Build history of the part. All positions in model axes, mm. A direction names the side the tool comes from. Round coordinates to 2 decimals unless told otherwise and drop trailing zeros. Write each loop counter-clockwise with the first axis right and the second up, starting at its lowest first coordinate (ties: lowest second). Pieces come first, ordered by that corner, then holes.
from build123d import *

# Parameters (mm, degrees)
SKETCH_1_W          = 135
SKETCH_1_H          = 80
EXTRUDE_1_DEPTH     = 60
CUT_EXTRUDE_START   = -1.5
CUT_EXTRUDE_1_DEPTH = 57
CUT_EXTRUDE_2_REACH = 170.003
SKETCH_4_R          = 23.5
SKETCH_5_W          = 135
SKETCH_5_H          = 15
EXTRUDE_2_DEPTH     = 5
M5_C_1_D            = 5.3
M5_C_1_DEPTH        = 5.2
M5_C_1_CBORE_D      = 11
M5_C_1_CBORE_DEPTH  = 0.5
M5_C_1_TIP          = 1.59228064
FILLET_1_R          = 5
FILLET_2_R          = 5
FILLET_3_R          = 5


with BuildPart() as part:
    # 草图1 → 凸台-拉伸1 (new body)
    with BuildSketch(Plane.XY):
        with Locations((67.5, -40)):
            Rectangle(SKETCH_1_W, SKETCH_1_H)
    extrude(amount=EXTRUDE_1_DEPTH)

    # 草图2 → 切除-拉伸1 (cut)
    with BuildSketch(Plane.XY.offset(60).offset(CUT_EXTRUDE_START)):
        Polygon((24.108601621, -76.68), (13.8, -76.68), (13.8, -19.68), (68.3, -19.68), (68.3, -76.68), align=None)
    extrude(amount=-CUT_EXTRUDE_1_DEPTH, mode=Mode.SUBTRACT)

    # 草图4 → 切除-拉伸2 (cut, up to next)
    with BuildSketch(Plane(origin=(135, 0, 0), x_dir=(0, 0, -1), z_dir=(1, 0, 0)), mode=Mode.PRIVATE) as cut_extrude_2_sk1:
        with Locations(Location((-30, -48.18, 0), (0, 0, 90))):
            Circle(SKETCH_4_R)
    cut_extrude_2_tool1 = extrude(cut_extrude_2_sk1.sketch, amount=-CUT_EXTRUDE_2_REACH, mode=Mode.PRIVATE) & part.part
    add(cut_extrude_2_tool1.solids().sort_by_distance((135, -48.18, 30))[0], mode=Mode.SUBTRACT)

    # 草图5 → 凸台-拉伸2 (add)
    with BuildSketch(Plane(origin=(0, 0, 0), x_dir=(1, 0, 0), z_dir=(0, 1, 0))):
        with Locations((67.5, 7.5)):
            Rectangle(SKETCH_5_W, SKETCH_5_H)
        with Locations((67.5, -67.5)):
            Rectangle(SKETCH_5_W, SKETCH_5_H)
    extrude(amount=-EXTRUDE_2_DEPTH)

    # M5 六角头螺栓C级的柱形沉头孔1
    with Locations(Plane(origin=(0, -5, 0), x_dir=(-1, 0, 0), z_dir=(0, -1, 0))):
        with Locations((-110, 7.5), (-25, 7.5), (-110, -67.5), (-25, -67.5)):
            CounterBoreHole(M5_C_1_D / 2, M5_C_1_CBORE_D / 2, M5_C_1_CBORE_DEPTH, depth=M5_C_1_DEPTH)
            with Locations((0, 0, -(M5_C_1_DEPTH + M5_C_1_TIP / 2))):  # 118° drill point
                Cone(0, M5_C_1_D / 2, M5_C_1_TIP, mode=Mode.SUBTRACT)

    # 圆角1
    fillet_1_edges = [part.edges().sort_by_distance(p)[0] for p in [
        (0, -42.5, 0),
        (0, -42.5, 60),
    ]]
    fillet(fillet_1_edges, radius=FILLET_1_R)

    # 圆角2
    fillet_2_edges = [part.edges().sort_by_distance(p)[0] for p in [
        (70, -80, 60),
        (70, -80, 0),
        (0, -80, 30),
        (1.464466094, -80, 1.464466094),
        (1.464466094, -80, 58.535533906),
    ]]
    fillet(fillet_2_edges, radius=FILLET_2_R)

    # 圆角3
    fillet_3_edges = [part.edges().sort_by_distance(p)[0] for p in [
        (0, -2.5, -15),
        (135, -2.5, -15),
        (135, -2.5, 75),
        (0, -2.5, 75),
    ]]
    fillet(fillet_3_edges, radius=FILLET_3_R)


solid = part.part
1) Slice it at D-D (y = -10). Write the cut outline in (x, z), plus the area to 3 significant figures.
Results:
outline: (0, 5) arc R5 ccw to (5, 0) - (135, 0) - (135, 60) - (5, 60) arc R5 ccw to (0, 55) - close
area: 8,090 mm2
2) Slice it at A-A (x = 110). Write the cut outline in (y, z), plus the area to 3 significant figures.
Results:
outline: (-80, 5) arc R5 ccw to (-75, 0) - (-5, 0) - (-5, -2) - (-4.5, -2) - (-4.5, -4.85) - (0, -4.85) - (0, 64.85) - (-4.5, 64.85) - (-4.5, 62) - (-5, 62) - (-5, 60) - (-75, 60) arc R5 ccw to (-80, 55) - close; (-5, -15) - (0, -15) - (0, -10.15) - (-4.5, -10.15) - (-4.5, -13) - (-5, -13) - close; (-5, 73) - (-4.5, 73) - (-4.5, 70.15) - (0, 70.15) - (0, 75) - (-5, 75) - close; hole circle Ø47 at (-48.18, 30)
area: 3,150 mm2
3) Which spindle directions (+Z, -Z, +X, -X, +Y, -Y) get a long thin tool onto all of the face, cutting with end or side? Do faces 1 (the flat face through (68.3, -73, 30)), 2 (the cylindrical face through (102.117, -25.765, 37.059)), 3 (the cylindrical face through (71, -78, 59)), 4 (the cylindrical face through (111.223, -2.218, -5.149)), 5 (the flat face through (113, -4.5, -6)). Say none if no direction does.
Results:
face 1: none
face 2: +X
face 3: +Z, +X, -X, -Y
face 4: +Y, -Y
face 5: -Y
4) Slice it at B-B (z = 67.5). Write the cut outline in (x, y).
Results:
outline: (0, -5) - (19.5, -5) - (19.5, -4.5) - (22.35, -4.5) - (22.35, 0) - (0, 0) - close; (27.65, -4.5) - (30.5, -4.5) - (30.5, -5) - (104.5, -5) - (104.5, -4.5) - (107.35, -4.5) - (107.35, 0) - (27.65, 0) - close; (112.65, -4.5) - (115.5, -4.5) - (115.5, -5) - (135, -5) - (135, 0) - (112.65, 0) - close
5) Wall check: L1, parallel to Z at x = 110, y = -4; L2, parallel to X at y = -4.6, z = 67.5; L3, parallel to Y at x = 40, z = 46.5. Give the ranges that are in metal, low to high.
Results:
L1: z = -15 to -10.15, -4.85 to 64.85, 70.15 to 75
L2: x = 0 to 19.5, 30.5 to 104.5, 115.5 to 135
L3: y = -80 to -76.68, -19.68 to 0
6) Pin check, flat tips, straight feed: pin 1 Ø21 at (x, y) = (45, -31.5) entering from +Z; pin 2 Ø10 at (x, z) = (101, -1.5) entering from -Y; pin 3 Ø10 at (x, z) = (110, 67.5) entering from -Y. Stop position of each tip, or through.
Results:
pin 1: stops at z = 60
pin 2: stops at y = -79.77
pin 3: stops at y = -4.5
7) Slice it at C-C (x = 96.5). Write the cut outline in (y, z), plus the area to 3 significant figures.
Results:
outline: (-80, 5) arc R5 ccw to (-75, 0) - (-5, 0) - (-5, -15) - (0, -15) - (0, 75) - (-5, 75) - (-5, 60) - (-75, 60) arc R5 ccw to (-80, 55) - close; hole circle Ø47 at (-48.18, 30)
area: 3,200 mm2
8) Mould opens along Z. For faces 6 (the cylindrical face through (24.43, -2.22, 70.09)), 7 (the flat face through (28, -4.5, -6)), 8 (the cylindrical face through (1, -3, -13)), 9 (the flat face through (135, -22, 31)) say: released by +Z, released by -Z, zero draft, split by the parting line, or undercut.
Results:
face 6: undercut
face 7: undercut
face 8: released by -Z
face 9: zero draft
